Could you check a few things on this model? Use its own coordinates, in mm. Face numbers are marked on the shaded views. A direction names the side the tool comes from. Coordinates: 2 decimals unless noted, no trailing zeros. Loops run counter-clockwise (first coordinate to the right, second up) from the corner with the lowest first, then second, coordinate; pieces in that order, holes last. Notation, with made-up numbers: (-35, -19.5) -> (-1, -19.5) arc R25 cw to (-1, -7.5) -> close; hole circle Ø4 at (79.5, -6.75). An arc over 180 degrees is marked (long way). One line per question, with ' | ' between items.
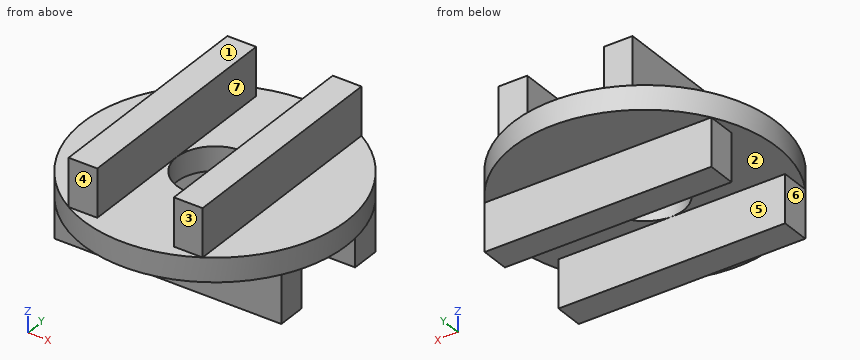
from build123d import *

# Parameters (mm, degrees)
SZKIC1_R                    = 55
SZKIC1_R_2                  = 16
DODANIE_WYCI_GNI_CIE1_DEPTH = 10
SZKIC2_W                    = 12
SZKIC2_H                    = 94.678403028
DODANIE_WYCI_GNI_CIE2_DEPTH = 20
SZKIC3_W                    = 94.678403028
SZKIC3_H                    = 12
DODANIE_WYCI_GNI_CIE3_DEPTH = 20


with BuildPart() as part:
    # Szkic1 → Dodanie-wyciągnięcie1 (new body)
    with BuildSketch(Plane.XY):
        Circle(SZKIC1_R)
        Circle(SZKIC1_R_2, mode=Mode.SUBTRACT)
    extrude(amount=DODANIE_WYCI_GNI_CIE1_DEPTH)

    # Szkic2 → Dodanie-wyciągnięcie2 (add)
    with BuildSketch(Plane.XY.offset(10)):
        with Locations((-22, 0)):
            Rectangle(SZKIC2_W, SZKIC2_H)
        with Locations((22, 0)):
            Rectangle(SZKIC2_W, SZKIC2_H)
    extrude(amount=DODANIE_WYCI_GNI_CIE2_DEPTH)

    # Szkic3 → Dodanie-wyciągnięcie3 (add)
    with BuildSketch(Plane(origin=(0, 0, 0), x_dir=(-1, 0, 0), z_dir=(0, 0, -1))):
        with Locations((0, -22)):
            Rectangle(SZKIC3_W, SZKIC3_H)
        with Locations((0, 22)):
            Rectangle(SZKIC3_W, SZKIC3_H)
    extrude(amount=DODANIE_WYCI_GNI_CIE3_DEPTH)


solid = part.part
1) I'm going to push flat-ended pins straight in: pin 1 Ø22 at (x, z) = (15.5, -7.5) entering from +Y; pin 2 Ø9.5 at (y, z) = (-20, -10.5) entering from -X; pin 3 Ø5 at (y, z) = (-11, 19.5) entering from -X. Where does each tip first touch, or does it pass through?
Data:
pin 1: y = 54.49 | pin 2: x = -47.34 | pin 3: x = -28
2) On a 3-axis mill with a long thin cutter (end or side, diameter ignored), from which of +Z, -Z, +X, -X, +Y, -Y can I reach the whole of each face in a straight line? I mean the marked faces 4, 5, 6 and 7. Say none if no direction works.
Data:
face 4: +Z, +X, -X, -Y | face 5: -Z, +X, -X | face 6: -Z, -X, +Y, -Y | face 7: +Z, +Y, -Y
3) If we section it at B-B on y = 14.5: Please give me the cut outline in (x, z).
Data:
outline: (-53.05, 0) -> (-6.76, 0) -> (-6.76, 10) -> (-16, 10) -> (-16, 30) -> (-28, 30) -> (-28, 10) -> (-53.05, 10) -> close; (6.76, 0) -> (53.05, 0) -> (53.05, 10) -> (28, 10) -> (28, 30) -> (16, 30) -> (16, 10) -> (6.76, 10) -> close
4) If we section it at D-D on y = -19: Please give me the cut outline in (x, z), and give its area (3 significant figures).
Data:
outline: (-51.61, 0) -> (-47.34, 0) -> (-47.34, -20) -> (47.34, -20) -> (47.34, 0) -> (51.61, 0) -> (51.61, 10) -> (28, 10) -> (28, 30) -> (16, 30) -> (16, 10) -> (-16, 10) -> (-16, 30) -> (-28, 30) -> (-28, 10) -> (-51.61, 10) -> close | area: 3,410 mm²
5) I need wall thicknesses on line 1 along X through (y, z) = (-45, 13); line 2 along X through (y, z) = (0, 4.5). Which ranges of each line are inside material? Lowest first, please. Write a range as from..to.
Data:
line 1: -28..-16, 16..28 | line 2: -55..-16, 16..55
6) If we section it at A-A on z = 21: Please give me the cut outline in (x, y).
Data:
outline: (-28, -47.34) -> (-16, -47.34) -> (-16, 47.34) -> (-28, 47.34) -> close; (16, -47.34) -> (28, -47.34) -> (28, 47.34) -> (16, 47.34) -> close
7) We'd pull the mould along Y, two halves only. Please class the marked faces 1, 2 and 3: pulls with the +Y half, pulls with the -Y half, needs draft (parallel to the pull), parting line crosses it, or undercut.
Data:
face 1: needs draft | face 2: undercut | face 3: pulls with the -Y half
8) If we section it at C-C on x = -11: Please give me the cut outline in (y, z), and give its area (3 significant figures).
Data:
outline: (-53.89, 0) -> (-28, 0) -> (-28, -20) -> (-16, -20) -> (-16, 0) -> (-11.62, 0) -> (-11.62, 10) -> (-53.89, 10) -> close; (11.62, 0) -> (16, 0) -> (16, -20) -> (28, -20) -> (28, 0) -> (53.89, 0) -> (53.89, 10) -> (11.62, 10) -> close | area: 1,330 mm²
